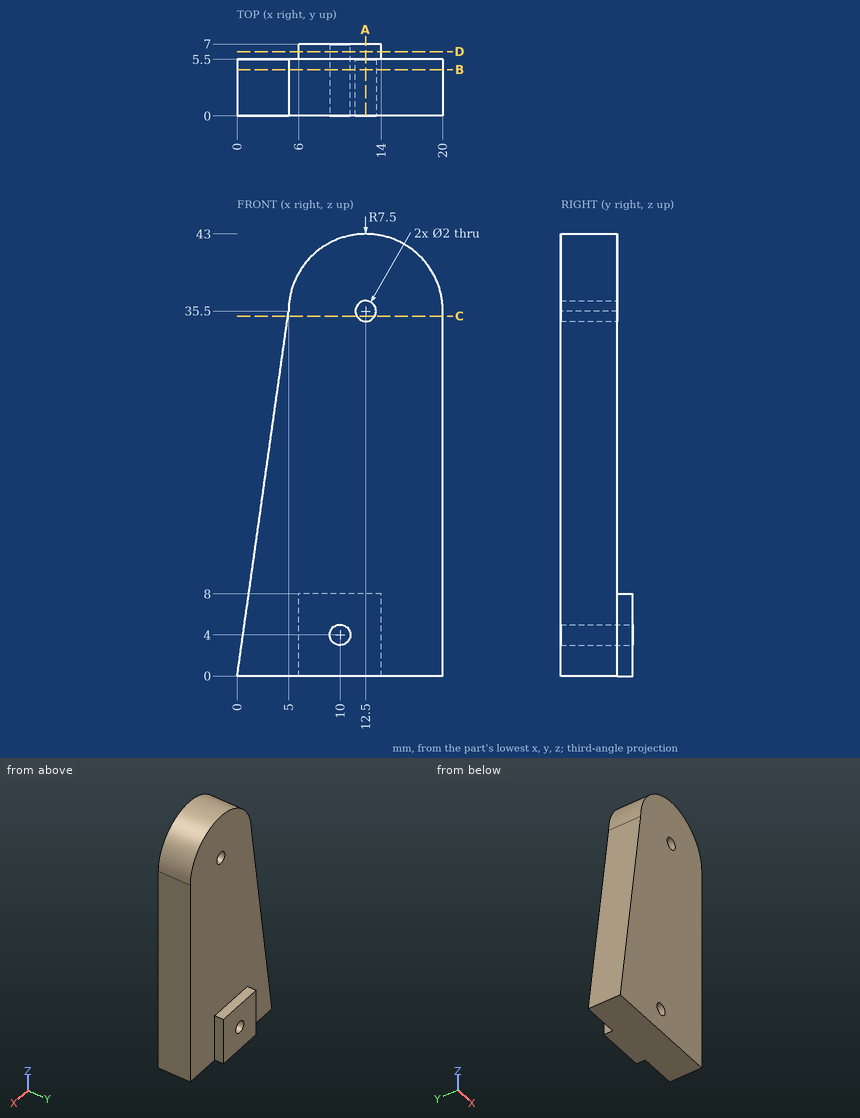
Could you check a few things on this drawing? It's one solid part, dimensions in mm from its lowest x, y, z. Round coordinates to 2 decimals unless told otherwise and drop trailing zeros. Order: outer loops, then holes, each group sorted by start corner. A loop starts at its lowest first (then second) coordinate and runs counter-clockwise, first axis right, second up. Notation, with made-up numbers: M 29.5,46 L 76.5,46 A15 cw 76.5,70 Z; hole C -20,10 d3. An arc over 180 degrees is marked long. One line per item, written item: value.
(1) I'm going to push flat-ended pins straight in: P1, Ø1.2, axis at x = 9, y = 6.5, coming from the +Z side; P2, Ø0.8, axis at y = 6.5, z = 4.5, coming from the +X side; P3, Ø3, axis at x = 13.5, z = 15, coming from the +Y side; P4, Ø1.2, axis at x = 10, z = 4, coming from the -Y side. Where does each tip first touch, or does it pass through?
Ans:
P1: stops at z = 8
P2: stops at x = 14
P3: stops at y = 5.5
P4: passes through
(2) Imagine slicing it at D-D (y = 6.25). Write out the boundary of the cut face in (x, z).
Ans:
outline: M 6,0 L 14,0 L 14,8 L 6,8 Z; hole C 10,4 d2
(3) Imagine slicing it at C-C (z = 35). Write out the boundary of the cut face in (x, y), and give its area (3 significant figures).
Ans:
outline: M 4.93,0 L 11.63,0 L 11.63,5.5 L 4.93,5.5 Z; M 13.37,0 L 20,0 L 20,5.5 L 13.37,5.5 Z
area: 73.4 mm^2
(4) I need wall thicknesses on line 1 along Z through (x, y) = (12.5, 1.45); line 2 along Y through (x, z) = (16.5, 16); line 3 along Z through (x, y) = (10, 2.75). Which ranges of each line are inside material? Lowest first, please. Write a range as from..to.
Ans:
line 1: z = 0..34.5, 36.5..43
line 2: y = 0..5.5
line 3: z = 0..3, 5..42.57
(5) Imagine slicing it at A-A (x = 12.5). Write out the boundary of the cut face in (y, z), and give its area (4 significant figures).
Ans:
outline: M 0,0 L 7,0 L 7,8 L 5.5,8 L 5.5,34.5 L 0,34.5 Z; M 0,36.5 L 5.5,36.5 L 5.5,43 L 0,43 Z
area: 237.5 mm^2
(6) Imagine slicing it at B-B (y = 4.5). Write out the boundary of the cut face in (x, z).
Ans:
outline: M 0,0 L 20,0 L 20,35.5 A7.5 ccw 5,35.5 Z; hole C 10,4 d2; hole C 12.5,35.5 d2
